```python
from build123d import *

# Parameters (mm, degrees)
SKETCH1_W           = 146
SKETCH1_H           = 146
BOSS_EXTRUDE1_DEPTH = 20
SKETCH2_R           = 63.5
BOSS_EXTRUDE2_DEPTH = 12.7
SKETCH3_R           = 65


with BuildPart() as part:
    # Sketch1 → Boss-Extrude1 (new body)
    with BuildSketch(Plane.XY):
        Rectangle(SKETCH1_W, SKETCH1_H)
    extrude(amount=BOSS_EXTRUDE1_DEPTH)

    # Sketch2 → Boss-Extrude2 (add)
    with BuildSketch(Plane(origin=(0, 0, 0), x_dir=(-1, 0, 0), z_dir=(0, 0, -1))):
        Circle(SKETCH2_R)
    extrude(amount=BOSS_EXTRUDE2_DEPTH)

    # Sweep1: sweep along a path in Sketch4
    with BuildLine(Plane(origin=(0, 0, 0), x_dir=(0, 0, -1), z_dir=(1, 0, 0))) as sweep1_path:
        Line((-20, 0), (-100, 0))
        Line((-100, 0), (-184.264888743, -70.706637066))
    # Sketch3 → Sweep1 (sweep)
    with BuildSketch(Plane.XY.offset(20)):
        Circle(SKETCH3_R)
    sweep(path=sweep1_path.line, transition=Transition.RIGHT)


solid = part.part
```
Input: part model. Units: mm. Frame: model coordinates. A direction names the side the tool comes from. Round coordinates to 2 decimals unless told otherwise and drop trailing zeros. Loops run counter-clockwise (first coordinate to the right, second up) from the corner with the lowest first, then second, coordinate; pieces in that order, holes last. Notation, with made-up numbers: (27.5, 17) -> (73.5, 17) arc R22 ccw to (73.5, 51) -> close; hole circle Ø1 at (60.25, 67). An arc over 180 degrees is marked (long way). Use one line per item in the form item = value. Start each with the question number.
Item 1: Section query A-A on x = 0. Return the cut outline in (y, z), then the cut area to 3 significant figures.
Item 2: Section query C-C on x = 41. Return the cut outline in (y, z).
Item 3: Set-up query: faces 1 (the face through (-66, 1, 20)), 2 (the face through (-1, -73, 10)), 3 (the face through (13.77, -61.99, -6.26)). Return all of +Z, -Z, +X, -X, +Y, -Y with unobstructed straight access to the full face (end or side cutting, diameter ignored); none if empty.
Item 4: Contact query for flat-ended pins moving along their axis: pin 1 Ø1 at (y, z) = (-22, 35) entering from +X; pin 2 Ø10 at (x, y) = (49, -75.5) entering from -Z; pin 3 Ø10 at (x, y) = (-12.5, -83) entering from +Z. Output: stop coordinate, or through.
Item 5: Mould query, pull axis Z, two halves, no side actions, for faces 4 (the face through (-8.46, 11.47, 186.59)), 5 (the face through (-1, 73, 10)), 6 (the face through (64, 1, 0)). Classes: pulls with the +Z half, pulls with the -Z half, needs draft (parallel to the pull), parting line crosses it, or undercut.
Item 6: Material intervals for L1, parallel to Z at x = -11.5, y = -71; L2, parallel to Z at x = 66, y = -13; L3, parallel to Z at x = 54, y = -48, sorted ascending. Write a range as from..to.
Item 7: Section query B-B on z = 24. Return the cut outline in (x, y).
Ans:
q1.outline = (-120.5, 142.48) -> (-65, 76.34) -> (-65, 20) -> (-73, 20) -> (-73, 0) -> (-63.5, 0) -> (-63.5, -12.7) -> (63.5, -12.7) -> (63.5, 0) -> (73, 0) -> (73, 20) -> (65, 20) -> (65, 123.66) -> (-20.91, 226.05) -> close
q1.area = 29,200 mm^2
q2.outline = (-109.34, 151.84) -> (-50.44, 81.64) -> (-50.44, 20) -> (-73, 20) -> (-73, 0) -> (-48.49, 0) -> (-48.49, -12.7) -> (48.49, -12.7) -> (48.49, 0) -> (73, 0) -> (73, 20) -> (50.44, 20) -> (50.44, 118.36) -> (-32.07, 216.69) -> close
q3.face_1 = none
q3.face_2 = -Z, +X, -X, -Y
q3.face_3 = -Z
q4.pin_1 = 61.34
q4.pin_2 = 0
q4.pin_3 = 178.15
q5.face_4 = undercut
q5.face_5 = needs draft
q5.face_6 = pulls with the -Z half
q6.L1 = 0..20, 85.09..184.02
q6.L2 = 0..20
q6.L3 = 0..20, 100.92..203.32
q7.outline = circle Ø130 at (0, 0)
